Check sheet for the drawn part. Datum: minimum x, y, z corner. Units: mm. Coordinates: 2 decimals unless noted, no trailing zeros. Write each loop counter-clockwise with the first axis right and the second up, starting at its lowest first coordinate (ties: lowest second). Pieces come first, ordered by that corner, then holes. Notation, with made-up numbers: (-23, -12.5) -> (0, -12.5) arc R34 cw to (0, 23.5) -> close; hole circle Ø10 at (8, -26). An arc over 180 degrees is marked (long way). Answer in a Markdown table with one row per item.
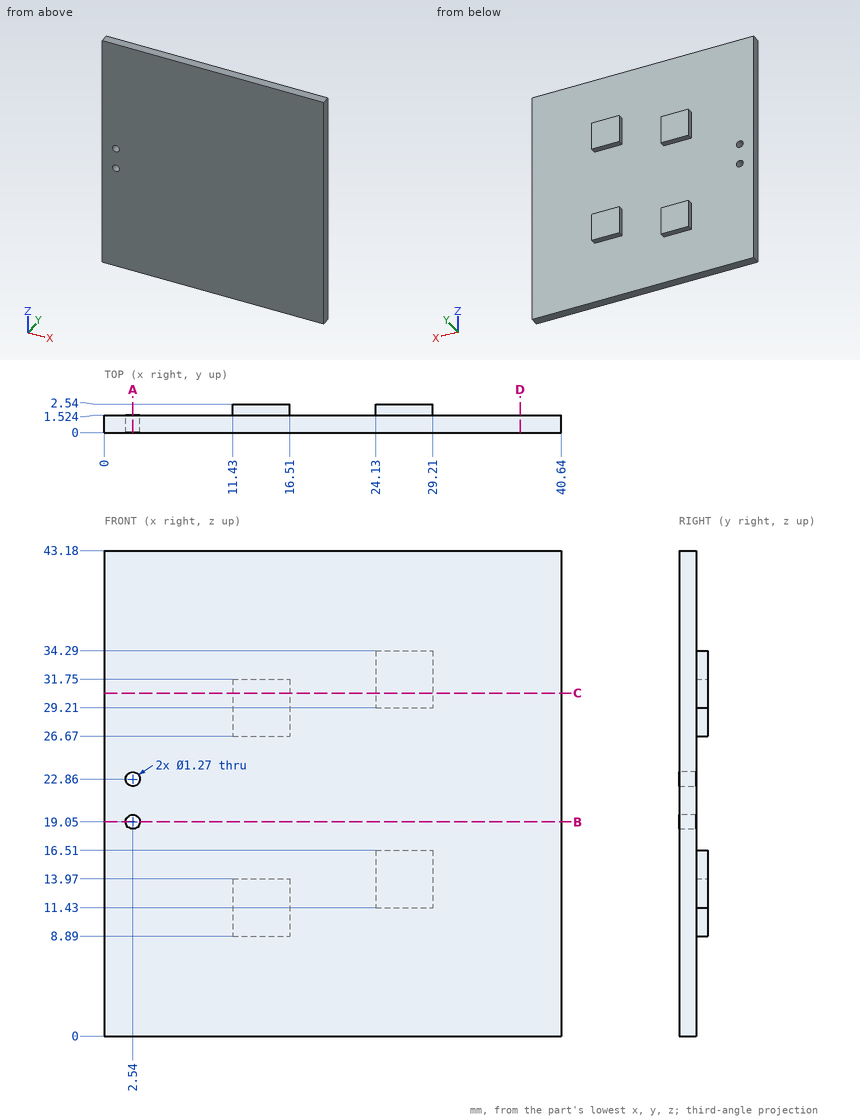
1. Sectioned sample at A-A, the plane x = 2.54. Record the cut outline in (y, z) (3 decimals).
Findings below:
| item | result |
|---|---|
| outline | (0, 0) -> (1.524, 0) -> (1.524, 18.415) -> (0, 18.415) -> close; (0, 19.685) -> (1.524, 19.685) -> (1.524, 22.225) -> (0, 22.225) -> close; (0, 23.495) -> (1.524, 23.495) -> (1.524, 43.18) -> (0, 43.18) -> close |
2. Go/stop test with flat-tipped pins: pin 1 (1.1 mm diameter, centred on x = 2.54, z = 19.05, fed in from -Y); pin 2 (0.5 mm diameter, centred on y = 2, z = 28, fed in from +X); pin 3 (0.5 mm diameter, centred on x = 26, y = 2, fed in from -Z); pin 4 (2 mm diameter, centred on x = 2.54, z = 22.86, fed in from +Y). Record where each tip stops, or that it passes through.
Findings below:
| item | result |
|---|---|
| pin 1 | passes through |
| pin 2 | stops at x = 16.51 |
| pin 3 | stops at z = 11.43 |
| pin 4 | stops at y = 1.52 |
3. Sectioned sample at B-B, the plane z = 19.05. Record the cut outline in (x, y) (3 decimals), and give its area (3 significant figures).
Findings below:
| item | result |
|---|---|
| outline | (0, 0) -> (1.905, 0) -> (1.905, 1.524) -> (0, 1.524) -> close; (3.175, 0) -> (40.64, 0) -> (40.64, 1.524) -> (3.175, 1.524) -> close |
| area | 60.0 mm² |
4. Sectioned sample at C-C, the plane z = 30.5. Record the cut outline in (x, y).
Findings below:
| item | result |
|---|---|
| outline | (0, 0) -> (40.64, 0) -> (40.64, 1.52) -> (29.21, 1.52) -> (29.21, 2.54) -> (24.13, 2.54) -> (24.13, 1.52) -> (16.51, 1.52) -> (16.51, 2.54) -> (11.43, 2.54) -> (11.43, 1.52) -> (0, 1.52) -> close |
5. Material ranges on probe 1 along X at (y, z) = (0.7, 19.05) (3 decimals); probe 2 along Z at (x, y) = (27, 1.6); probe 3 along Y at (x, z) = (3, 7), recorded low to high. Write a range as from..to.
Findings below:
| item | result |
|---|---|
| probe 1 | x = 0..1.905, 3.175..40.64 |
| probe 2 | z = 11.43..16.51, 29.21..34.29 |
| probe 3 | y = 0..1.52 |
6. Sectioned sample at D-D, the plane x = 37. Record the cut outline in (y, z).
Findings below:
| item | result |
|---|---|
| outline | (0, 0) -> (1.52, 0) -> (1.52, 43.18) -> (0, 43.18) -> close |
